Could you check a few things on this model? Use its own coordinates, in mm. Round coordinates to 2 decimals unless told otherwise and drop trailing zeros. Loops run counter-clockwise (first coordinate to the right, second up) from the corner with the lowest first, then second, coordinate; pieces in that order, holes last. Notation, with made-up numbers: (-7, 49) -> (5, 49) arc R14 ccw to (5, 75) -> close; hole circle Ø3 at (81, -2). An arc over 180 degrees is marked (long way). Write each question's results on one line, items separated by ' | '. Start each with the question number.
1) We'd pull the mould along Y, two halves only. Please class faces 1 (the cylindrical face through (0, -2, -7)), 2 (the cylindrical face through (-0.867, -3.905, -7.398)), 3 (the flat face through (2, -2, -15)): pulls with the +Y half, pulls with the -Y half, needs draft (parallel to the pull), parting line crosses it, or undercut.
2) Imagine slicing it at A-A, the plane x = 0. List the corners of the cut face in (y, z) for me.
3) For P1, Ø1.5, axis at y = -2.5, z = -3.5, coming from the +X side; P2, Ø2, axis at y = -3, z = -4, coming from the -X side; P3, Ø3, axis at x = -2.5, z = -4, coming from the +Y side, each with a flat end and sliding along its axis, tell me the tip position at first contact or that it passes through.
4) If I drill on probe 1 along Y at (x, z) = (0, -4.5); probe 2 along X at (y, z) = (-0.25, -13.75); probe 3 along Y at (x, z) = (-1.75, -2.75), over which ranges is the centre line in solid material (lowest first)?
5) Imagine slicing it at C-C, the plane z = -5.25. List the corners of the cut face in (x, y) for me, plus the area to 3 significant figures.
from build123d import *

# Parameters (mm, degrees)
SKETCH_1_R      = 4
SKETCH_1_R_2    = 2
EXTRUDE_1_DEPTH = 15
FILLET_1_R      = 0.2


with BuildPart() as part:
    # 草图1 → 凸台-拉伸1 (new body)
    with BuildSketch(Plane.XY):
        Circle(SKETCH_1_R)
        Circle(SKETCH_1_R_2, mode=Mode.SUBTRACT)
    extrude(amount=-EXTRUDE_1_DEPTH)

    # 圆角1
    fillet_1_edges = [part.edges().sort_by_distance(p)[0] for p in [
        (-4, 0, 0),
        (-4, 0, -15),
        (-2, 0, -15),
        (-2, 0, 0),
    ]]
    fillet(fillet_1_edges, radius=FILLET_1_R)


solid = part.part
Checked values:
1) face 1: undercut | face 2: parting line crosses it | face 3: needs draft
2) outline: (-4, -14.8) arc R0.2 ccw to (-3.8, -15) -> (-2.2, -15) arc R0.2 ccw to (-2, -14.8) -> (-2, -0.2) arc R0.2 ccw to (-2.2, 0) -> (-3.8, 0) arc R0.2 ccw to (-4, -0.2) -> close; (2, -14.8) arc R0.2 ccw to (2.2, -15) -> (3.8, -15) arc R0.2 ccw to (4, -14.8) -> (4, -0.2) arc R0.2 ccw to (3.8, 0) -> (2.2, 0) arc R0.2 ccw to (2, -0.2) -> close
3) P1: x = 3.6 | P2: x = -3.46 | P3: y = 3.87
4) probe 1: -4 to -2, 2 to 4 | probe 2: -3.99 to -1.98, 1.98 to 3.99 | probe 3: -3.6 to -0.97, 0.97 to 3.6
5) outline: circle Ø8 at (0, 0); hole circle Ø4 at (0, 0) | area: 37.7 mm^2
